Can you work these out from the model? Positions are in its coordinate system, mm. A direction names the side the tool comes from. Coordinates: 2 decimals unless noted, no trailing zeros. Loops run counter-clockwise (first coordinate to the right, second up) from the corner with the lowest first, then second, coordinate; pieces in that order, holes last. Notation, with made-up numbers: (36, -31) -> (57, -31) arc R26 cw to (57, 5) -> close; hole circle Ø9 at (12, 73.5). An arc over 180 degrees is marked (long way). Put each result on its own line as item: value. Start each with the question number.
Item 1: Please list where these lines run through material, in increasing order: L1, parallel to X at y = 49, z = 15.25; L2, parallel to Y at x = 104, z = 1.5; L3, parallel to X at y = 37, z = 1.5. Write a range as from..to.
Item 2: If we section it at D-D on y = 83: Please give me the cut outline in (x, z), plus the area to 3 significant figures.
Item 3: Will these pins go through, and if not, where does the flat tip stop? P1, Ø10, axis at x = 66.5, y = 19.5, coming from the +Z side; P2, Ø1.2, axis at x = 103.5, y = 14.5, coming from the -Z side.
Item 4: If we section it at B-B on z = 10.5: Please give me the cut outline in (x, y), plus the area to 3 significant figures.
Item 5: If we section it at A-A on x = 50: Please give me the cut outline in (y, z), plus the area to 3 significant figures.
Item 6: For faces 1 (the cylindrical face through (14, 23, 13)), 2 (the flat face through (150, 41, 0)), 3 (the flat face through (39, 41, 3)), which set-ups out of +Z, -Z, +X, -X, +Y, -Y let a thin tool reach every point of the face, with its end or its side?
Item 7: If we section it at C-C on y = 50: State how many separate pieces and enclosed holes the cut face has, plus the area to 3 significant figures.
Item 8: We'd pull the mould along X, two halves only. Please class faces 4 (the flat face through (0, 49, 9)), 5 (the flat face through (99, 0, 9)), 6 (the flat face through (200, 49, 9)), 7 (the cylindrical face through (47.42, 52.365, 4.056)): pulls with the +X half, pulls with the -X half, needs draft (parallel to the pull), parting line crosses it, or undercut.
```python
from build123d import *

# Parameters (mm, degrees)
SKETCH1_W           = 200
SKETCH1_H           = 100
BOSS_EXTRUDE1_DEPTH = 18.5
SKETCH2_R           = 45
CUT_EXTRUDE1_DEPTH  = 10.5
SKETCH3_R           = 3.5
CUT_EXTRUDE2_DEPTH  = 19.5
CUT_EXTRUDE4_DEPTH  = 3
CUT_EXTRUDE5_DEPTH  = 2


with BuildPart() as part:
    # Sketch1 → Boss-Extrude1 (new body)
    with BuildSketch(Plane.XY):
        with Locations((100, 50)):
            Rectangle(SKETCH1_W, SKETCH1_H)
    extrude(amount=BOSS_EXTRUDE1_DEPTH)

    # Sketch2 → Cut-Extrude1 (cut)
    with BuildSketch(Plane.XY.offset(18.5)):
        with Locations((50, 50)):
            Circle(SKETCH2_R)
        with Locations((150, 50)):
            Circle(SKETCH2_R)
    extrude(amount=-CUT_EXTRUDE1_DEPTH, mode=Mode.SUBTRACT)

    # Sketch3 → Cut-Extrude2 (cut, through all)
    with BuildSketch(Plane.XY.offset(18.5)):
        with Locations((50, 50)):
            Circle(SKETCH3_R)
        with Locations((150, 50)):
            Circle(SKETCH3_R)
    extrude(amount=-CUT_EXTRUDE2_DEPTH, mode=Mode.SUBTRACT)

    # Sketch4 → Cut-Extrude4 (cut)
    with BuildSketch(Plane(origin=(0, 0, 0), x_dir=(-1, 0, 0), z_dir=(0, 0, -1))):
        with BuildLine():
            Line((-133.600331897, 55.296115572), (-133.600331897, 25.39429873))
            ThreePointArc((-133.600331897, 25.39429873), (-150, 8.994630628), (-166.399668103, 25.39429873))
            Line((-166.399668103, 25.39429873), (-166.399668103, 55.296115572))
            ThreePointArc((-166.399668103, 55.296115572), (-150, 71.695783675), (-133.600331897, 55.296115572))
        make_face()
        with BuildLine():
            Line((-141.600331897, 55.296115572), (-141.600331897, 25.39429873))
            ThreePointArc((-141.600331897, 25.39429873), (-150, 16.994630628), (-158.399668103, 25.39429873))
            Line((-158.399668103, 25.39429873), (-158.399668103, 55.296115572))
            ThreePointArc((-158.399668103, 55.296115572), (-150, 63.695783675), (-141.600331897, 55.296115572))
        make_face(mode=Mode.SUBTRACT)
        with BuildLine():
            Line((-33.600331897, 55.296115572), (-33.600331897, 25.39429873))
            ThreePointArc((-33.600331897, 25.39429873), (-50, 8.994630628), (-66.399668103, 25.39429873))
            Line((-66.399668103, 25.39429873), (-66.399668103, 55.296115572))
            ThreePointArc((-66.399668103, 55.296115572), (-50, 71.695783675), (-33.600331897, 55.296115572))
        make_face()
        with BuildLine():
            Line((-41.600331897, 55.296115572), (-41.600331897, 25.39429873))
            ThreePointArc((-41.600331897, 25.39429873), (-50, 16.994630628), (-58.399668103, 25.39429873))
            Line((-58.399668103, 25.39429873), (-58.399668103, 55.296115572))
            ThreePointArc((-58.399668103, 55.296115572), (-50, 63.695783675), (-41.600331897, 55.296115572))
        make_face(mode=Mode.SUBTRACT)
    extrude(amount=-CUT_EXTRUDE4_DEPTH, mode=Mode.SUBTRACT)

    # Sketch5 → Cut-Extrude5 (cut)
    with BuildSketch(Plane(origin=(0, 0, 0), x_dir=(-1, 0, 0), z_dir=(0, 0, -1))):
        with BuildLine():
            Line((-110.1200005, 32.2499995), (-89.8000005, 32.2499995))
            ThreePointArc((-89.8000005, 32.2499995), (-87.8000005, 30.2499995), (-89.8000005, 28.2499995))
            Line((-89.8000005, 28.2499995), (-110.1200005, 28.2499995))
            ThreePointArc((-110.1200005, 28.2499995), (-112.1200005, 30.2499995), (-110.1200005, 32.2499995))
        make_face()
        with BuildLine():
            Line((-110.1200005, 16.9999995), (-89.8000005, 16.9999995))
            ThreePointArc((-89.8000005, 16.9999995), (-87.8000005, 14.9999995), (-89.8000005, 12.9999995))
            Line((-89.8000005, 12.9999995), (-110.1200005, 12.9999995))
            ThreePointArc((-110.1200005, 12.9999995), (-112.1200005, 14.9999995), (-110.1200005, 16.9999995))
        make_face()
    extrude(amount=-CUT_EXTRUDE5_DEPTH, mode=Mode.SUBTRACT)


solid = part.part
```
Solutions:
1. L1: 0..5.01, 94.99..105.01, 194.99..200
1. L2: 0..13, 17..28.25, 32.25..100
1. L3: 0..33.6, 41.6..58.4, 66.4..133.6, 141.6..158.4, 166.4..200
2. outline: (0, 0) -> (200, 0) -> (200, 18.5) -> (180.59, 18.5) -> (180.59, 8) -> (119.41, 8) -> (119.41, 18.5) -> (80.59, 18.5) -> (80.59, 8) -> (19.41, 8) -> (19.41, 18.5) -> (0, 18.5) -> close
2. area: 2,420 mm^2
3. P1: z = 8
3. P2: z = 2
4. outline: (0, 0) -> (200, 0) -> (200, 100) -> (0, 100) -> close; hole circle Ø90 at (50, 50); hole circle Ø90 at (150, 50)
4. area: 7,280 mm^2
5. outline: (0, 0) -> (8.99, 0) -> (8.99, 3) -> (16.99, 3) -> (16.99, 0) -> (46.5, 0) -> (46.5, 8) -> (5, 8) -> (5, 18.5) -> (0, 18.5) -> close; (53.5, 0) -> (63.7, 0) -> (63.7, 3) -> (71.7, 3) -> (71.7, 0) -> (100, 0) -> (100, 18.5) -> (95, 18.5) -> (95, 8) -> (53.5, 8) -> close
5. area: 801 mm^2
6. face 1: +Z
6. face 2: -Z, +X, -X, +Y, -Y
6. face 3: -Z
7. separate pieces: 3
7. enclosed holes: 0
7. area: 1,600 mm^2
8. face 4: pulls with the -X half
8. face 5: needs draft
8. face 6: pulls with the +X half
8. face 7: undercut
